Model file for the job. Use its own axes, mm. A direction names the side the tool comes from. Coordinates: 2 decimals unless noted, no trailing zeros. Write each loop counter-clockwise with the first axis right and the second up, starting at its lowest first coordinate (ties: lowest second). Pieces come first, ordered by that corner, then holes. Notation, with made-up numbers: (42, 6) -> (86, 6) arc R21 cw to (86, 44) -> close; hole circle Ø1 at (-29, 9.5). An arc over 180 degrees is marked (long way). Write item = value, one per line. Start each with the question number.
from build123d import *

# Parameters (mm, degrees)
F0_R     = 12.5
F0_R_2   = 8
F1_DEPTH = 44
F2_R     = 15
F2_R_2   = 12.5
F3_DEPTH = 10
F4_SIZE  = 0.5


with BuildPart() as f1:
    # F0 (on Front) → F1 (new body)
    with BuildSketch(Plane.XZ):
        Circle(F0_R)
        Circle(F0_R_2, mode=Mode.SUBTRACT)
    extrude(amount=-F1_DEPTH)

    # F2 (on Front) → F3 (join)
    with BuildSketch(Plane.XZ):
        Circle(F2_R)
        Circle(F2_R_2, mode=Mode.SUBTRACT)
    extrude(amount=-F3_DEPTH)

    # F4
    f4_edges = [f1.edges().sort_by_distance(p)[0] for p in [
        (-8, 0, 0),
        (-15, 0, 0),
        (-15, 10, 0),
        (-12.5, 44, 0),
        (-8, 44, 0),
    ]]
    chamfer(f4_edges, length=F4_SIZE)


solid = f1.part
(1) Saw through at C-C (y = 16). Give the cut face in (x, z), then the cut area to 3 significant figures.
(2) Drop flat-ended pins along their axis: pin 1 Ø8.5 at (x, z) = (4, 1) entering from +Y; pin 2 Ø2 at (y, z) = (17, 9) entering from +X; pin 3 Ø1.5 at (x, y) = (-11.5, 34) entering from +Z; pin 4 Ø9.5 at (x, z) = (0, 0) entering from -Y. Give the stop position or say it passes through.
(3) 3-axis set-ups, long thin cutter, end or side, ignore diameter. For faces 4 (the face through (-8.2, 44, 2.8)), 5 (the face through (11.923, 26.516, 3.755)): which of +Z, -Z, +X, -X, +Y, -Y reach the whole face in a straight line?
(4) Mould opens along X. For faces 1 (the face through (-11, 10, 7)), 2 (the face through (-14.985, 4.937, 0.66)), 3 (the face through (-1.73, 21.7, -7.81)) say: released by +X, released by -X, zero draft, split by the parting line, or undercut.
(5) Drill centre lines: line 1 along Z through (x, y) = (0, 19); line 2 along X through (y, z) = (24, -5) (3 decimals); line 3 along Z through (x, y) = (-7.25, 5). Where is each one in solid material? Low to high.
(6) Saw through at A-A (z = 0). Give the cut face in (x, y), then the cut area to 3 significant figures.
(7) Saw through at D-D (y = 8.5). Give the cut face in (x, z), then the cut area to 3 significant figures.
(8) Saw through at B-B (x = 0). Give the cut face in (y, z).
Returned:
q1.outline = circle Ø25 at (0, 0); hole circle Ø16 at (0, 0)
q1.area = 290 mm2
q2.pin_1 = 43.87
q2.pin_2 = 9.6
q2.pin_3 = 6.38
q2.pin_4 = through
q3.face_4 = +Z, -Z, +X, -X, +Y
q3.face_5 = +Y
q4.face_1 = zero draft
q4.face_2 = split by the parting line
q4.face_3 = undercut
q5.line_1 = -12.5 to -8, 8 to 12.5
q5.line_2 = -11.456 to -6.245, 6.245 to 11.456
q5.line_3 = -13.13 to -3.38, 3.38 to 13.13
q6.outline = (-15, 0.5) -> (-14.5, 0) -> (-8.5, 0) -> (-8, 0.5) -> (-8, 43.5) -> (-8.5, 44) -> (-12, 44) -> (-12.5, 43.5) -> (-12.5, 10) -> (-14.5, 10) -> (-15, 9.5) -> close; (8, 0.5) -> (8.5, 0) -> (14.5, 0) -> (15, 0.5) -> (15, 9.5) -> (14.5, 10) -> (12.5, 10) -> (12.5, 43.5) -> (12, 44) -> (8.5, 44) -> (8, 43.5) -> close
q6.area = 445 mm2
q7.outline = circle Ø30 at (0, 0); hole circle Ø16 at (0, 0)
q7.area = 506 mm2
q8.outline = (0, -14.5) -> (0.5, -15) -> (9.5, -15) -> (10, -14.5) -> (10, -12.5) -> (43.5, -12.5) -> (44, -12) -> (44, -8.5) -> (43.5, -8) -> (0.5, -8) -> (0, -8.5) -> close; (0, 8.5) -> (0.5, 8) -> (43.5, 8) -> (44, 8.5) -> (44, 12) -> (43.5, 12.5) -> (10, 12.5) -> (10, 14.5) -> (9.5, 15) -> (0.5, 15) -> (0, 14.5) -> close
